```python
from build123d import *

# Parameters (mm, degrees)
F0_W     = 2
F0_H     = 4
F4_R     = 5
F5_R     = 4
F6_DEPTH = 25
F7_R     = 1.99999


# Not quite as in the source:
# - a fillet or chamfer is up to 0.001 mm smaller than in the source, because OpenCascade refuses the exact size
# - a feature names something its author has since deleted; it is built from what else it names


with BuildPart() as f1:
    # F0 (on Right) → F1 (revolve)
    with BuildSketch(Plane.YZ):
        with Locations((-26, 6)):
            Rectangle(F0_W, F0_H)
        Polygon((-29, 0), (-25, 0), (-25, 2), (-25, 4), (-27, 4), (-29, 4), align=None)
        Polygon((-25, 2), (-25, 0), (-23.256576216, 0), (0, -6.0669329259), (0, -4), (-23, 2), align=None)
    revolve(axis=Axis((0, 0, 1), (0, 0, 1)))

    # F2 (on Right) → F3 (revolve)
    with BuildSketch(Plane.YZ):
        Polygon((-10, -8), (-6, -8), (-6, -12), (0, -12), (0, -4), (-10, -1.3913043478), align=None)
    revolve(axis=Axis((0, 0, -8), (0, 0, 1)))

    # F4
    f4_edges = [f1.edges().sort_by_distance(p)[0] for p in [
        (0, 10, -3.458237),
    ]]
    fillet(f4_edges, radius=F4_R)

    # F5 (on Top) → F6 (cut)
    with BuildSketch(Plane.XY):
        Circle(F5_R)
    extrude(amount=-F6_DEPTH, mode=Mode.SUBTRACT)

    # F7 (radius 2 in the source; OpenCascade refuses exactly that, so slightly less here)
    f7_edges = [f1.edges().sort_by_distance(p)[0] for p in [
        (0, 27, 4),
    ]]
    fillet(f7_edges, radius=F7_R)


solid = f1.part
```
Build history of the part. All positions in model axes, mm. A direction names the side the tool comes from. Give positions to 0.01 mm unless a question says otherwise; leave off trailing zeros. Loops run counter-clockwise (first coordinate to the right, second up) from the corner with the lowest first, then second, coordinate; pieces in that order, holes last.
1) Band-saw the part on B-B on z = -1.25. List the corners of the cut face in (x, y), then the cut area to 3 significant figures.
Values follow:
outline: circle Ø36.93 at (0, 0); hole circle Ø21.08 at (0, 0)
area: 722 mm2
2) Drop flat-ended pins along their axis: P1, Ø2, axis at x = -5.5, y = 5, coming from the +Z side; P2, Ø5, axis at y = -5.5, z = 1, coming from the -X side; P3, Ø6, axis at x = 8.5, z = 5, coming from the -Y side; P4, Ø7, axis at x = 0, y = 0, coming from the -Z side. Give the stop position or say it passes through.
Values follow:
P1: stops at z = -1.8
P2: stops at x = -28.84
P3: stops at y = -28.44
P4: passes through
3) Probe line 1 along X through (y, z) = (0, -10); line 2 along X through (y, z) = (0, 3.4); line 3 along Z through (x, y) = (-7, -26). List the from-to ranges inside material, lowest first.
Values follow:
line 1: x = -6 to -4, 4 to 6
line 2: x = -29 to -25, 25 to 29
line 3: z = 0 to 8
4) Band-saw the part on A-A on z = -10.5. List the corners of the cut face in (x, y), then the cut area to 3 significant figures.
Values follow:
outline: circle Ø12 at (0, 0); hole circle Ø8 at (0, 0)
area: 62.8 mm2
5) Two-plate mould, pull along X, no slides. Class faces 4 (the face through (-5.065, 1.125, -2.646)), 5 (the face through (-3.92, 1.42, -12)), 6 (the face through (-26.36, 5.85, 7.01)): released by +X, released by -X, zero draft, split by the parting line, or undercut.
Values follow:
face 4: undercut
face 5: zero draft
face 6: split by the parting line
6) 3-axis set-ups, long thin cutter, end or side, ignore diameter. For faces 1 (the face through (9, 22, 0)), 2 (the face through (-8, -24, 8)), 3 (the face through (7.509, -23.846, 5.042)): which of +Z, -Z, +X, -X, +Y, -Y reach the whole face in a straight line?
Values follow:
face 1: -Z
face 2: +Z, +X, -X, +Y, -Y
face 3: +Z
